```python
from build123d import *

# Parameters (mm, degrees)
SKETCH_1_R               = 28
SKETCH_1_R_2             = 2.6
EXTRUDE_1_DEPTH          = 12
CUT_EXTRUDE_2_DEPTH      = 1
CUT_EXTRUDE_2_DEPTH_BACK = 13


with BuildPart() as part:
    # 草图1 → 凸台-拉伸1 (new body)
    with BuildSketch(Plane(origin=(0, 0, 0), x_dir=(1, 0, 0), z_dir=(0, 1, 0))):
        Circle(SKETCH_1_R)
        with Locations((10.5, 18.186533479)):
            Circle(SKETCH_1_R_2, mode=Mode.SUBTRACT)
        with Locations((21, 0)):
            Circle(SKETCH_1_R_2, mode=Mode.SUBTRACT)
        with Locations((10.5, -18.186533479)):
            Circle(SKETCH_1_R_2, mode=Mode.SUBTRACT)
        with Locations((-10.5, -18.186533479)):
            Circle(SKETCH_1_R_2, mode=Mode.SUBTRACT)
        with Locations((-21, 0)):
            Circle(SKETCH_1_R_2, mode=Mode.SUBTRACT)
        with Locations((-10.5, 18.186533479)):
            Circle(SKETCH_1_R_2, mode=Mode.SUBTRACT)
    extrude(amount=EXTRUDE_1_DEPTH)

    # 草图4 → 切除-拉伸2 (cut, two sides)
    with BuildSketch(Plane(origin=(0, 12, 0), x_dir=(1, 0, 0), z_dir=(0, 1, 0))) as cut_extrude_2_sk:
        with BuildLine():
            ThreePointArc((4.758569662, 16.444127766), (7.500000636, 12.99038069), (11.861748987, 12.343106429))
            ThreePointArc((11.861748987, 12.343106429), (17.297017892, 9.986437089), (16.620317219, 4.10102167))
            ThreePointArc((16.620317219, 4.10102167), (15, -7.34e-07), (16.620318223, -4.101022742))
            ThreePointArc((16.620318223, -4.101022742), (17.297017158, -9.98643836), (11.861747557, -12.343106096))
            ThreePointArc((11.861747557, -12.343106096), (7.499999364, -12.990381424), (4.758569235, -16.444129171))
            ThreePointArc((4.758569235, -16.444129171), (-7.34e-07, -19.972875449), (-4.758569662, -16.444127766))
            ThreePointArc((-4.758569662, -16.444127766), (-7.500000636, -12.99038069), (-11.861748987, -12.343106429))
            ThreePointArc((-11.861748987, -12.343106429), (-17.297017892, -9.986437089), (-16.620317219, -4.10102167))
            ThreePointArc((-16.620317219, -4.10102167), (-15, 7.34e-07), (-16.620318223, 4.101022742))
            ThreePointArc((-16.620318223, 4.101022742), (-17.297017158, 9.98643836), (-11.861747557, 12.343106096))
            ThreePointArc((-11.861747557, 12.343106096), (-7.499999364, 12.990381424), (-4.758569235, 16.444129171))
            ThreePointArc((-4.758569235, 16.444129171), (7.34e-07, 19.972875449), (4.758569662, 16.444127766))
        make_face()
    extrude(amount=CUT_EXTRUDE_2_DEPTH, mode=Mode.SUBTRACT)
    extrude(cut_extrude_2_sk.sketch, amount=-CUT_EXTRUDE_2_DEPTH_BACK, mode=Mode.SUBTRACT)


solid = part.part
```
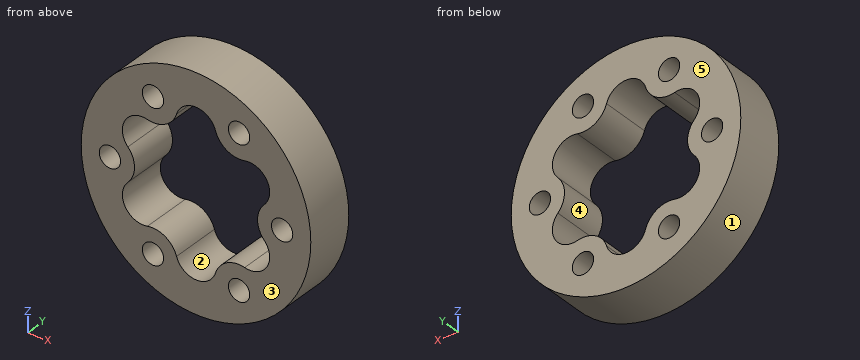
For this review, take the finished solid that the model builds, in its own axes (mm). Face numbers are marked on the shaded views. A direction names the side the tool comes from. Coordinates: 2 decimals unless noted, no trailing zeros. Loops run counter-clockwise (first coordinate to the right, second up) from the corner with the lowest first, then second, coordinate; pieces in that order, holes last.
1. Add section C-C, the plane y = 6.25. Give the boundary of the cut face in (x, z).
2. Add section A-A, the plane x = -21. Give the boundary of the cut face in (y, z).
3. For line 1 (X direction, y = 8.75, z = 0); line 2 (Z direction, x = 12, y = 1.5); line 3 (Z direction, x = 10.5, y = 6.5), list the stretches that pass through material, from the lowest coordinate up.
4. For the marked faces 4 and 5, list the 3-axis set-ups (+Z, -Z, +X, -X, +Y, -Y) from which the entire face can be reached by the end or side of a thin tool; tool diameter is ignored.
5. Add section D-D, the plane x = -10.5. Give the boundary of the cut face in (y, z).
6. Mouldability with a two-part tool opening along X and no side actions: class the marked faces 1, 2 and 3 as +X half, -X half, draft (parallel to the pull), parting line (faces both ways), or undercut.
7. Insertion check: P1, Ø6, axis at x = 10.5, z = 18.19, coming from the -Y side; P2, Ø4, axis at x = 10.5, z = -18.19, coming from the +Y side; P3, Ø1.5, axis at y = 10, z = -4, coming from the -X side; P4, Ø1.5, axis at y = 5, z = -14.5, coming from the -X side. Each pin has a flat end and moves straight along its axis. Give the tip position at first contact, or say it passes through.
8. Add section B-B, the plane z = -9. Give the boundary of the cut face in (x, y), then the cut area to 3 significant figures.
Result:
1. outline: circle Ø56 at (0, 0); hole circle Ø5.2 at (-21, 0); hole (-16.62, -4.1) arc R4.97 ccw to (-11.86, -12.34) arc R6 cw to (-4.76, -16.44) arc R4.97 ccw to (4.76, -16.44) arc R6 cw to (11.86, -12.34) arc R4.97 ccw to (16.62, -4.1) arc R6 cw to (16.62, 4.1) arc R4.97 ccw to (11.86, 12.34) arc R6 cw to (4.76, 16.44) arc R4.97 ccw to (-4.76, 16.44) arc R6 cw to (-11.86, 12.34) arc R4.97 ccw to (-16.62, 4.1) arc R6 cw to start; hole circle Ø5.2 at (-10.5, -18.19); hole circle Ø5.2 at (-10.5, 18.19); hole circle Ø5.2 at (10.5, -18.19); hole circle Ø5.2 at (10.5, 18.19); hole circle Ø5.2 at (21, 0)
2. outline: (0, -18.52) - (12, -18.52) - (12, -2.6) - (0, -2.6) - close; (0, 2.6) - (12, 2.6) - (12, 18.52) - (0, 18.52) - close
3. line 1: x = -28 to -23.6, -18.4 to -15, 15 to 18.4, 23.6 to 28
3. line 2: z = -25.3 to -20.31, -16.06 to -12.37, 12.37 to 16.06, 20.31 to 25.3
3. line 3: z = -25.96 to -20.79, -15.59 to -12.19, 12.19 to 15.59, 20.79 to 25.96
4. face 4: +Y, -Y
4. face 5: +Z, -Z, +X, -X, +Y
5. outline: (0, -25.96) - (12, -25.96) - (12, -20.79) - (0, -20.79) - close; (0, -15.59) - (12, -15.59) - (12, -12.19) - (0, -12.19) - close; (0, 12.19) - (12, 12.19) - (12, 15.59) - (0, 15.59) - close; (0, 20.79) - (12, 20.79) - (12, 25.96) - (0, 25.96) - close
6. face 1: parting line
6. face 2: undercut
6. face 3: draft
7. P1: stops at y = 0
7. P2: passes through
7. P3: stops at x = -27.81
7. P4: stops at x = -24.39
8. outline: (-26.51, 0) - (-17.73, 0) - (-17.73, 12) - (-26.51, 12) - close; (17.73, 0) - (26.51, 0) - (26.51, 12) - (17.73, 12) - close
8. area: 211 mm2
